Input: part model. Units: mm. Frame: model coordinates. Face numbers are marked on the shaded views. A direction names the side the tool comes from. Coordinates: 2 decimals unless noted, no trailing zeros. Write each loop counter-clockwise with the first axis right and the second up, starting at its lowest first coordinate (ties: lowest second). Pieces come first, ordered by that corner, then holes. Notation, with made-up numbers: M 8,72.5 L 35,72.5 A23 ccw 35,94.5 Z; hole C -7,11 d9. An arc over 180 degrees is marked long. Use CSV: the item, a comma, the result in double quotes.
```python
from build123d import *

# Parameters (mm, degrees)
SKETCH4_R          = 9.0551
SKETCH4_R_2        = 8.89635
CUT_EXTRUDE2_DEPTH = 7.112
CUT_EXTRUDE1_DEPTH = 7.112
CIRPATTERN1_COUNT  = 28


with BuildPart() as part:
    # Sketch1 → Revolve1 (revolve)
    with BuildSketch(Plane.XY, mode=Mode.PRIVATE) as revolve1_sk:
        with BuildLine():
            Line((-8.7376, 3.175), (8.7376, 3.175))
            Line((8.7376, 3.175), (8.7376, 11.176))
            Line((8.7376, 11.176), (7.7343, 11.176))
            ThreePointArc((7.7343, 11.176), (7.003726949, 10.549537058), (6.731, 9.6266))
            Line((6.731, 9.6266), (6.731, 9.0551))
            Line((6.731, 9.0551), (-0.381, 9.0551))
            Line((-0.381, 9.0551), (-0.381, 9.6266))
            ThreePointArc((-0.381, 9.6266), (-0.653726949, 10.549537058), (-1.3843, 11.176))
            Line((-1.3843, 11.176), (-2.3876, 11.176))
            Line((-2.3876, 11.176), (-2.3876, 8.7376))
            Line((-2.3876, 8.7376), (-8.7376, 8.7376))
            Line((-8.7376, 8.7376), (-8.7376, 3.175))
        make_face()
    revolve(revolve1_sk.sketch.rotate(Axis((-8.7376, 0, 0), (1, 0, 0)), 90), axis=Axis((-8.7376, 0, 0), (1, 0, 0)))

    # Sketch4 → Cut-Extrude2 (cut)
    with BuildSketch(Plane(origin=(-0.381, 0, 0), x_dir=(0, 0, -1), z_dir=(1, 0, 0))):
        Circle(SKETCH4_R)
        Circle(SKETCH4_R_2, mode=Mode.SUBTRACT)
    extrude(amount=CUT_EXTRUDE2_DEPTH, mode=Mode.SUBTRACT)

    # Sketch3 → Cut-Extrude1 (cut)
    with BuildSketch(Plane(origin=(-0.381, 0, 0), x_dir=(0, 0, -1), z_dir=(1, 0, 0))):
        with BuildLine():
            Line((-0.643388094, 8.873054439), (-0.340062676, 8.222570981))
            Line((-0.340062676, 8.222570981), (0.340062676, 8.222570981))
            Line((0.340062676, 8.222570981), (0.643388094, 8.873054439))
            ThreePointArc((0.643388094, 8.873054439), (0, 8.89635), (-0.643388094, 8.873054439))
        make_face()
    cut_extrude1 = extrude(amount=CUT_EXTRUDE1_DEPTH, mode=Mode.SUBTRACT)

    # CirPattern1: Cut-Extrude1 ×28 about axis
    cirpattern1_axis = Axis((0, 0, 0), (1, 0, 0))
    for i in range(1, CIRPATTERN1_COUNT):
        add(cut_extrude1.rotate(cirpattern1_axis, i * 360 / CIRPATTERN1_COUNT), mode=Mode.SUBTRACT)


solid = part.part
```
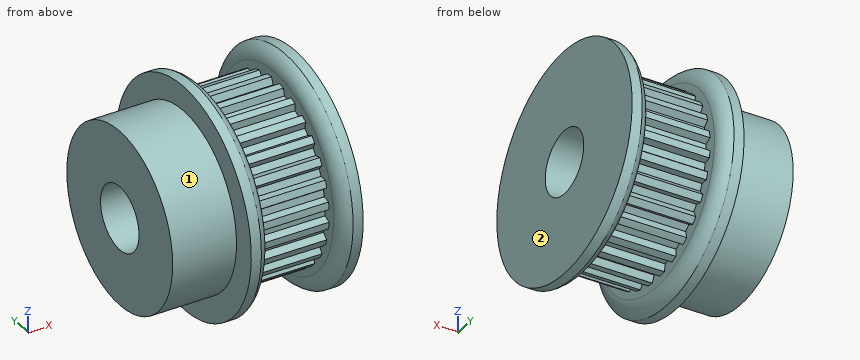
1. Contact query for flat-ended pins moving along their axis: pin 1 Ø11 at (y, z) = (-1, -2) entering from -X; pin 2 Ø4 at (x, z) = (-7, -0.5) entering from -Y; pin 3 Ø4 at (x, y) = (-6.5, 5) entering from +Z; pin 4 Ø5 at (x, y) = (-4, -6) entering from +Z. Output: stop coordinate, or through.
Resolved:
pin 1,"stops at x = -8.74"
pin 2,"stops at y = -8.74"
pin 3,"stops at z = 8.21"
pin 4,"stops at z = 10.4"
2. Access query for the marked faces 1 and 2. Directions: +Z, -Z, +X, -X, +Y, -Y. A direction counts if a zero-diameter tool reaches every point of the face in a straight line with its end or side. Return the directions, or none.
Resolved:
face 1,"-X"
face 2,"+Z, -Z, +X, +Y, -Y"
3. Section C-C (x = -4). Return loops of the section in (y, z) (3 decimals), then the cut area to 3 significant figures.
Resolved:
outline,"C 0,0 d17.475; hole C 0,0 d6.35"
area,"208 mm^2"
4. Material intervals for line 1 (X direction, y = -9, z = 0.5); line 2 (Y direction, x = -4.5, z = 0) (3 decimals); line 3 (Y direction, x = 1.5, z = 0) (3 decimals), sorted ascending. Write a range as [from, to].
Resolved:
line 1,"x = [-2.39, -0.38], [6.73, 8.74]"
line 2,"y = [-8.738, -3.175], [3.175, 8.738]"
line 3,"y = [-8.223, -3.175], [3.175, 8.223]"
5. Section D-D (x = -1.75). Return loops of the section in (y, z) (3 decimals).
Resolved:
outline,"C 0,0 d22.352; hole C 0,0 d6.35"
6. Section A-A (y = 0). Return loops of the section in (x, z) (3 decimals).
Resolved:
outline,"M -8.738,-8.738 L -2.388,-8.738 L -2.388,-11.176 L -1.384,-11.176 A1.698 ccw -0.381,-9.627 L -0.381,-8.223 L 6.731,-8.223 L 6.731,-9.627 A1.698 ccw 7.734,-11.176 L 8.738,-11.176 L 8.738,-3.175 L -8.738,-3.175 Z; M -8.738,3.175 L 8.738,3.175 L 8.738,11.176 L 7.734,11.176 A1.698 ccw 6.731,9.627 L 6.731,8.223 L -0.381,8.223 L -0.381,9.627 A1.698 ccw -1.384,11.176 L -2.388,11.176 L -2.388,8.738 L -8.738,8.738 Z"
